Verification items for the finished model (mm, model axes). A direction names the side the tool comes from. Give positions to 0.01 mm unless a question says otherwise; leave off trailing zeros. Order: outer loops, then holes, each group sorted by start corner. A loop starts at its lowest first (then second) coordinate and runs counter-clockwise, first axis right, second up. Notation, with made-up numbers: (13.5, -8) -> (29.5, -8) arc R20 ccw to (29.5, 6) -> close; hole circle Ø10 at (16.5, -28). An arc over 180 degrees is marked (long way). One line per question, with ' | ' between items. Start each with the question number.
Q1. Material ranges on probe 1 along X at (y, z) = (31, -2.25); probe 2 along Y at (x, z) = (170, -2); probe 3 along Y at (x, z) = (13, -6.5), recorded low to high. Write a range as [from, to].
Q2. Access from +Z, -Z, +X, -X, +Y, -Y to the whole of each face (thin tool, end or side, straight path). Record for faces 1 (the cylindrical face through (164.1, 36.4, -2.7)), 2 (the cylindrical face through (129.15, 53.01, -4.93)).
Q3. Section check C-C on x = 170. Record the cut outline in (y, z), plus the area to 3 significant figures.
Q4. Section check A-A on x = 60.5. Record the cut outline in (y, z), plus the area to 3 significant figures.
Q5. Go/stop test with flat-tipped pins: pin 1 (6.5 mm diameter, centred on x = 108, y = 5, fed in from -Z); pin 2 (5 mm diameter, centred on x = 171.5, y = 29, fed in from +Z). Record where each tip stops, or that it passes through.
Q6. Section check D-D on z = -7.25. Give the number of separate pieces and of enclosed holes in the cut face, plus the area to 3 significant figures.
Q7. Mould release check, pull along X, two halves, no side actions. Record for faces 3 (the flat face through (132, 70, -5)), 4 (the cylindrical face through (9.479, 41.966, -4.93)), 5 (the cylindrical face through (101.05, 34.19, -4.93)), 6 (the flat face through (126, 47, 0)): released by +X, released by -X, zero draft, split by the parting line, or undercut.
Q8. Section check B-B on y = 5. Record the cut outline in (x, z).
from build123d import *

# Parameters (mm, degrees)
CROQUIS1_R              = 8
SALIENTE_EXTRUIR1_DEPTH = 10
CROQUIS2_R              = 2.05
CORTAR_EXTRUIR1_DEPTH   = 240.3491174
SALIENTE_EXTRUIR2_START = -4.5
CROQUIS3_R              = 8
CROQUIS3_R_2            = 4
SALIENTE_EXTRUIR2_DEPTH = 4.5
CROQUIS4_R              = 4
CORTAR_EXTRUIR2_DEPTH   = 240.3491174


with BuildPart() as part:
    # Croquis1 → Saliente-Extruir1 (new body)
    with BuildSketch(Plane.XY):
        with BuildLine():
            Line((0, 0), (208, 0))
            Line((208, 0), (208, 80))
            ThreePointArc((208, 80), (170, 118), (132, 80))
            Line((132, 80), (132, 60))
            ThreePointArc((132, 60), (129.071067812, 52.928932188), (122, 50))
            Line((122, 50), (10, 50))
            ThreePointArc((10, 50), (2.928932188, 47.071067812), (0, 40))
            Line((0, 40), (0, 0))
        make_face()
        with Locations((170, 80)):
            Circle(CROQUIS1_R, mode=Mode.SUBTRACT)
        with Locations((170, 31)):
            Circle(CROQUIS1_R, mode=Mode.SUBTRACT)
    extrude(amount=-SALIENTE_EXTRUIR1_DEPTH)

    # Croquis2 → Cortar-Extruir1 (cut, through all)
    with BuildSketch(Plane(origin=(0, 0, -10), x_dir=(-1, 0, 0), z_dir=(0, 0, -1))):
        with Locations((-203, 5)):
            Circle(CROQUIS2_R)
        with Locations((-155.5, 5)):
            Circle(CROQUIS2_R)
        with Locations((-108, 5)):
            Circle(CROQUIS2_R)
        with Locations((-60.5, 5)):
            Circle(CROQUIS2_R)
        with Locations((-13, 5)):
            Circle(CROQUIS2_R)
    extrude(amount=-CORTAR_EXTRUIR1_DEPTH, mode=Mode.SUBTRACT)

    # Croquis3 → Saliente-Extruir2 (add)
    with BuildSketch(Plane(origin=(0, 0, -10), x_dir=(-1, 0, 0), z_dir=(0, 0, -1)).offset(SALIENTE_EXTRUIR2_START)):
        with Locations(Location((-170, 31, 0), (0, 0, 180))):
            Circle(CROQUIS3_R)
        with Locations((-170, 31)):
            Circle(CROQUIS3_R_2, mode=Mode.SUBTRACT)
    extrude(amount=SALIENTE_EXTRUIR2_DEPTH)

    # Croquis4 → Cortar-Extruir2 (cut, through all)
    with BuildSketch(Plane.XY):
        with Locations((198, 31.490486181)):
            Circle(CROQUIS4_R)
        with Locations((104, 31.490486181)):
            Circle(CROQUIS4_R)
        with Locations((10, 38)):
            Circle(CROQUIS4_R)
    extrude(amount=-CORTAR_EXTRUIR2_DEPTH, mode=Mode.SUBTRACT)


solid = part.part
Filled in:
1) probe 1: [0, 100.03], [107.97, 162], [178, 194.03], [201.97, 208] | probe 2: [0, 23], [39, 72], [88, 118] | probe 3: [0, 2.95], [7.05, 35.35], [40.65, 50]
2) face 1: +Z | face 2: +Z, -Z, -X, +Y
3) outline: (0, -10) -> (27, -10) -> (27, -5.5) -> (23, -5.5) -> (23, 0) -> (0, 0) -> close; (35, -10) -> (72, -10) -> (72, 0) -> (39, 0) -> (39, -5.5) -> (35, -5.5) -> close; (88, -10) -> (118, -10) -> (118, 0) -> (88, 0) -> close | area: 896 mm²
4) outline: (0, -10) -> (2.95, -10) -> (2.95, 0) -> (0, 0) -> close; (7.05, -10) -> (50, -10) -> (50, 0) -> (7.05, 0) -> close | area: 459 mm²
5) pin 1: z = -10 | pin 2: z = -5.5
6) separate pieces: 1 | enclosed holes: 10 | area: 14,500 mm²
7) face 3: released by -X | face 4: undercut | face 5: undercut | face 6: zero draft
8) outline: (0, -10) -> (10.95, -10) -> (10.95, 0) -> (0, 0) -> close; (15.05, -10) -> (58.45, -10) -> (58.45, 0) -> (15.05, 0) -> close; (62.55, -10) -> (105.95, -10) -> (105.95, 0) -> (62.55, 0) -> close; (110.05, -10) -> (153.45, -10) -> (153.45, 0) -> (110.05, 0) -> close; (157.55, -10) -> (200.95, -10) -> (200.95, 0) -> (157.55, 0) -> close; (205.05, -10) -> (208, -10) -> (208, 0) -> (205.05, 0) -> close
